from build123d import *

# Parameters (mm, degrees)
SKETCH1_W               = 55
SKETCH1_H               = 15
BOSS_EXTRUDE1_DEPTH     = 27
CUT_EXTRUDE1_DEPTH      = 42.355168964
CUT_EXTRUDE1_DEPTH_BACK = 42.355168964
SKETCH2_R               = 4.875
SKETCH4_W               = 15
SKETCH4_H               = 15
CUT_EXTRUDE2_DEPTH      = 22
CUT_EXTRUDE3_DEPTH      = 37.006943775
CUT_EXTRUDE3_DEPTH_BACK = 37.006943775
SKETCH5_R               = 1.5
FILLET1_R               = 2
FILLET2_R               = 7


with BuildPart() as part:
    # Sketch1 → Boss-Extrude1 (new body)
    with BuildSketch(Plane(origin=(0, 0, 0), x_dir=(1, 0, 0), z_dir=(0, 1, 0))):
        Rectangle(SKETCH1_W, SKETCH1_H)
    extrude(amount=BOSS_EXTRUDE1_DEPTH)

    # Sketch2 → Cut-Extrude1 (cut, two sides: drawn at the far end of the back side and taken through both)
    with BuildSketch(Plane.XY.offset(7.5).offset(-CUT_EXTRUDE1_DEPTH_BACK)):
        with Locations((0, 17.5)):
            Circle(SKETCH2_R)
    extrude(amount=CUT_EXTRUDE1_DEPTH + CUT_EXTRUDE1_DEPTH_BACK, mode=Mode.SUBTRACT)

    # Sketch4 → Cut-Extrude2 (cut)
    with BuildSketch(Plane(origin=(0, 27, 0), x_dir=(1, 0, 0), z_dir=(0, 1, 0))):
        with Locations((-20, 0)):
            Rectangle(SKETCH4_W, SKETCH4_H)
        with Locations((20, 0)):
            Rectangle(SKETCH4_W, SKETCH4_H)
    extrude(amount=-CUT_EXTRUDE2_DEPTH, mode=Mode.SUBTRACT)

    # Sketch5 → Cut-Extrude3 (cut, two sides: drawn at the far end of the back side and taken through both)
    with BuildSketch(Plane(origin=(0, 5, 0), x_dir=(1, 0, 0), z_dir=(0, 1, 0)).offset(-CUT_EXTRUDE3_DEPTH_BACK)):
        with Locations(Location((-20, 0, 0), (0, 0, 270))):
            Circle(SKETCH5_R)
        with Locations(Location((20, 0, 0), (0, 0, 270))):
            Circle(SKETCH5_R)
    extrude(amount=CUT_EXTRUDE3_DEPTH + CUT_EXTRUDE3_DEPTH_BACK, mode=Mode.SUBTRACT)

    # Fillet1
    fillet1_edges = [part.edges().sort_by_distance(p)[0] for p in [
        (-27.5, 5, 0),
        (-12.5, 5, 0),
        (27.5, 5, 0),
        (12.5, 5, 0),
    ]]
    fillet(fillet1_edges, radius=FILLET1_R)

    # Fillet2
    fillet2_edges = [part.edges().sort_by_distance(p)[0] for p in [
        (-12.5, 27, 0),
        (12.5, 27, 0),
    ]]
    fillet(fillet2_edges, radius=FILLET2_R)


solid = part.part
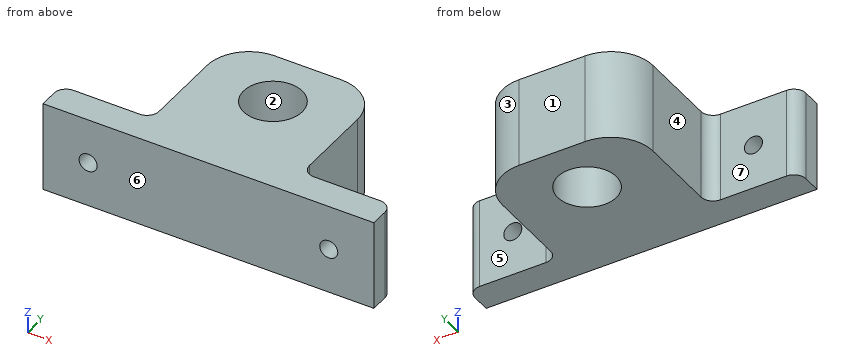
Check sheet for the modelled part. Datum: model origin and axes. Units: mm. Face numbers are marked on the shaded views. A direction names the side the tool comes from. Give positions to 0.01 mm unless a question says otherwise; leave off trailing zeros. Loops run counter-clockwise (first coordinate to the right, second up) from the corner with the lowest first, then second, coordinate; pieces in that order, holes last. Notation, with made-up numbers: M -38.75,51 L -23.75,51 A30 ccw -23.75,79 Z; hole C 3.5,49 d1. An arc over 180 degrees is marked long. Answer as a JSON object with one key per item and string values. Group by question number.
Q1. Cross-section at C-C on z = 0. Record the cut outline in (x, y) (3 decimals).
Q2. Cross-section at D-D on z = 6.5. Record the cut outline in (x, y) (3 decimals), then the cut area to 3 significant figures.
Q3. Cross-section at B-B on y = 17.5. Record the cut outline in (x, z) (3 decimals).
Q4. Go/stop test with flat-tipped pins: P1, Ø2, axis at y = 21.5, z = 0, coming from the +X side; P2, Ø9, axis at x = -20, z = -1.5, coming from the +Y side; P3, Ø9, axis at x = 18.5, z = 2, coming from the +Y side. Record where each tip stops, or that it passes through.
Q5. Cross-section at A-A on x = 0. Record the cut outline in (y, z) (3 decimals).
Q6. Release check for a two-part mould opening along X. For the marked faces 1, 2, 3 and 4 record: released by +X, released by -X, zero draft, split by the parting line, or undercut.
Q7. Material ranges on line 1 along X through (y, z) = (1.4, 0); line 2 along X through (y, z) = (17.5, -3.5) (3 decimals); line 3 along Z through (x, y) = (-20, 2.55), recorded low to high. Write a range as [from, to].
Q8. Access from +Z, -Z, +X, -X, +Y, -Y to the whole of each face (thin tool, end or side, straight path). Record for the marked faces 5, 6 and 7.
Evaluation:
{
 "1": {"outline": "M -27.5,0 L -21.5,0 L -21.5,5 L -25.5,5 A2 ccw -27.5,3 Z; M -18.5,0 L 18.5,0 L 18.5,5 L 14.5,5 A2 cw 12.5,7 L 12.5,20 A7 ccw 5.5,27 L -5.5,27 A7 ccw -12.5,20 L -12.5,7 A2 cw -14.5,5 L -18.5,5 Z; M 21.5,0 L 27.5,0 L 27.5,3 A2 ccw 25.5,5 L 21.5,5 Z; hole C 0,17.5 d9.75"},
 "2": {"outline": "M -27.5,0 L 27.5,0 L 27.5,3 A2 ccw 25.5,5 L 14.5,5 A2 cw 12.5,7 L 12.5,20 A7 ccw 5.5,27 L -5.5,27 A7 ccw -12.5,20 L -12.5,7 A2 cw -14.5,5 L -25.5,5 A2 ccw -27.5,3 Z; hole C 0,17.5 d9.75", "area": "729 mm2"},
 "3": {"outline": "M -12.5,-7.5 L -4.875,-7.5 L -4.875,7.5 L -12.5,7.5 Z; M 4.875,-7.5 L 12.5,-7.5 L 12.5,7.5 L 4.875,7.5 Z"},
 "4": {"P1": "stops at x = 12.48", "P2": "stops at y = 5", "P3": "stops at y = 5.06"},
 "5": {"outline": "M 0,-7.5 L 12.625,-7.5 L 12.625,7.5 L 0,7.5 Z; M 22.375,-7.5 L 27,-7.5 L 27,7.5 L 22.375,7.5 Z"},
 "6": {"face 1": "zero draft", "face 2": "undercut", "face 3": "released by +X", "face 4": "released by -X"},
 "7": {"line 1": "x = [-27.5, -21.5], [-18.5, 18.5], [21.5, 27.5]", "line 2": "x = [-12.5, -4.875], [4.875, 12.5]", "line 3": "z = [-7.5, -1.5], [1.5, 7.5]"},
 "8": {"face 5": "+Z, -Z, +X, +Y", "face 6": "+Z, -Z, +X, -X, -Y", "face 7": "+Z, -Z, -X, +Y"}
}
